Check sheet for the modelled part. Datum: model origin and axes. Units: mm. A direction names the side the tool comes from. Round coordinates to 2 decimals unless told otherwise and drop trailing zeros. Order: outer loops, then holes, each group sorted by start corner. A loop starts at its lowest first (then second) coordinate and runs counter-clockwise, first axis right, second up. Notation, with made-up numbers: M -12,36.25 L 28,36.25 A31 cw 28,74.25 Z; hole C 35,22.25 d3. An arc over 180 degrees is marked long. One line per item, written item: value. Start each with the question number.
(1) Cross-section at B-B, the plane y = 16. Enter the section's corners in (x, z), and give its area (3 significant figures).
(2) Cross-section at A-A, the plane x = 16.5. Enter the section's corners in (y, z), and give its area (3 significant figures).
(3) Release check for a two-part mould opening along X. For faces 4 (the face through (-25.5, 0, 1)), 5 (the face through (6, 20, 1)), 6 (the face through (-24, 20, 1)) record: released by +X, released by -X, zero draft, split by the parting line, or undercut.
(4) Depth check by flat-ended pin: pin 1 Ø0.9 at (x, z) = (24, 1) entering from -Y; pin 2 Ø1.5 at (y, z) = (-16.5, 2) entering from +X; pin 3 Ø1.5 at (x, z) = (-7.5, 2) entering from +Y. Enter the tip coordinate at first touch or a pass-through.
(5) Access from +Z, -Z, +X, -X, +Y, -Y to the whole of each face (thin tool, end or side, straight path). Record for faces 1 (the face through (24, -3, 1)), 2 (the face through (-18, 20, 1)), 3 (the face through (-24, 3, 1)).
(6) Thickness scan on L1, parallel to Y at x = -8, z = 1; L2, parallel to X at y = -3.5, z = 0.4. Record the ranges inside material, lowest first.
from build123d import *

# Parameters (mm, degrees)
SKETCH1_W               = 45
SKETCH1_H               = 40
BOSS_EXTRUDE1_DEPTH     = 3
SKETCH2_W               = 3
SKETCH2_H               = 6
BOSS_EXTRUDE2_DEPTH     = 3
LPATTERN1_COUNT         = 2
LPATTERN1_PITCH         = 12
LPATTERN1_COL_COUNT     = 2
LPATTERN1_COL_PITCH     = 12
SKETCH3_W               = 6
SKETCH3_H               = 3
BOSS_EXTRUDE3_DEPTH     = 3
LPATTERN2_COUNT         = 3
LPATTERN2_PITCH         = 12
LPATTERN2_COL_COUNT     = 3
LPATTERN2_COL_PITCH     = 12
SKETCH6_W               = 1.5
SKETCH6_H               = 3
CUT_EXTRUDE2_DEPTH      = 3
MIRROR1_COPY_1_SKETCH_W = 3
MIRROR1_COPY_1_SKETCH_H = 6
MIRROR1_COPY_1_DEPTH    = 3
MIRROR1_COPY_2_SKETCH_W = 3
MIRROR1_COPY_2_SKETCH_H = 6
MIRROR1_COPY_2_DEPTH    = 3


with BuildPart() as part:
    # Sketch1 → Boss-Extrude1 (new body)
    with BuildSketch(Plane.XY):
        Rectangle(SKETCH1_W, SKETCH1_H)
    extrude(amount=BOSS_EXTRUDE1_DEPTH)

    # Sketch2 → Boss-Extrude2 (add)
    with BuildSketch(Plane.ZY.offset(22.5)):
        with Locations((1.5, 0)):
            Rectangle(SKETCH2_W, SKETCH2_H)
    boss_extrude2 = extrude(amount=BOSS_EXTRUDE2_DEPTH)

    # LPattern1: Boss-Extrude2 ×2
    with Locations(*[(0, -i * LPATTERN1_PITCH, 0) for i in range(1, LPATTERN1_COUNT)]):
        add(boss_extrude2)

    # LPattern1 col: Boss-Extrude2 ×2
    with Locations(*[(0, i * LPATTERN1_COL_PITCH, 0) for i in range(1, LPATTERN1_COL_COUNT)]):
        add(boss_extrude2)

    # Sketch3 → Boss-Extrude3 (add)
    with BuildSketch(Plane(origin=(0, 20, 0), x_dir=(1, 0, 0), z_dir=(0, 1, 0))):
        with Locations((0, -1.5)):
            Rectangle(SKETCH3_W, SKETCH3_H)
    boss_extrude3 = extrude(amount=BOSS_EXTRUDE3_DEPTH)

    # LPattern2: Boss-Extrude3 ×3
    with Locations(*[(-i * LPATTERN2_PITCH, 0, 0) for i in range(1, LPATTERN2_COUNT)]):
        add(boss_extrude3)

    # LPattern2 col: Boss-Extrude3 ×3
    with Locations(*[(i * LPATTERN2_COL_PITCH, 0, 0) for i in range(1, LPATTERN2_COL_COUNT)]):
        add(boss_extrude3)

    # Sketch6 → Cut-Extrude2 (cut)
    with BuildSketch(Plane(origin=(0, 23, 0), x_dir=(1, 0, 0), z_dir=(0, 1, 0))):
        with Locations((26.25, -1.5)):
            Rectangle(SKETCH6_W, SKETCH6_H)
    cut_extrude2 = extrude(amount=-CUT_EXTRUDE2_DEPTH, mode=Mode.SUBTRACT)

    # Mirror1: Boss-Extrude2 across plane
    add(boss_extrude2.mirror(Plane(origin=(0, 0, 0), x_dir=(0, 0, 1), z_dir=(1, 0, 0))))

    # Mirror1 copy 1 sketch → Mirror1 copy 1 (add)
    with BuildSketch(Plane(origin=(22.5, -12, 0), x_dir=(0, 0, 1), z_dir=(1, 0, 0))):
        with Locations((1.5, 0)):
            Rectangle(MIRROR1_COPY_1_SKETCH_W, MIRROR1_COPY_1_SKETCH_H)
    extrude(amount=MIRROR1_COPY_1_DEPTH)

    # Mirror1 copy 2 sketch → Mirror1 copy 2 (add)
    with BuildSketch(Plane(origin=(22.5, 12, 0), x_dir=(0, 0, 1), z_dir=(1, 0, 0))):
        with Locations((1.5, 0)):
            Rectangle(MIRROR1_COPY_2_SKETCH_W, MIRROR1_COPY_2_SKETCH_H)
    extrude(amount=MIRROR1_COPY_2_DEPTH)

    # Mirror2: Cut-Extrude2 across plane
    add(cut_extrude2.mirror(Plane(origin=(0, 0, 0), x_dir=(0, 0, 1), z_dir=(1, 0, 0))), mode=Mode.SUBTRACT)


solid = part.part
Values found:
1. outline: M -22.5,0 L 22.5,0 L 22.5,3 L -22.5,3 Z
1. area: 135 mm^2
2. outline: M -20,0 L 20,0 L 20,3 L -20,3 Z
2. area: 120 mm^2
3. face 4: released by -X
3. face 5: undercut
3. face 6: zero draft
4. pin 1: y = -15
4. pin 2: x = 22.5
4. pin 3: y = 20
5. face 1: +Z, -Z, +X
5. face 2: +Z, -Z, +Y
5. face 3: +Z, -Z, -X
6. L1: -20 to 20
6. L2: -22.5 to 22.5
